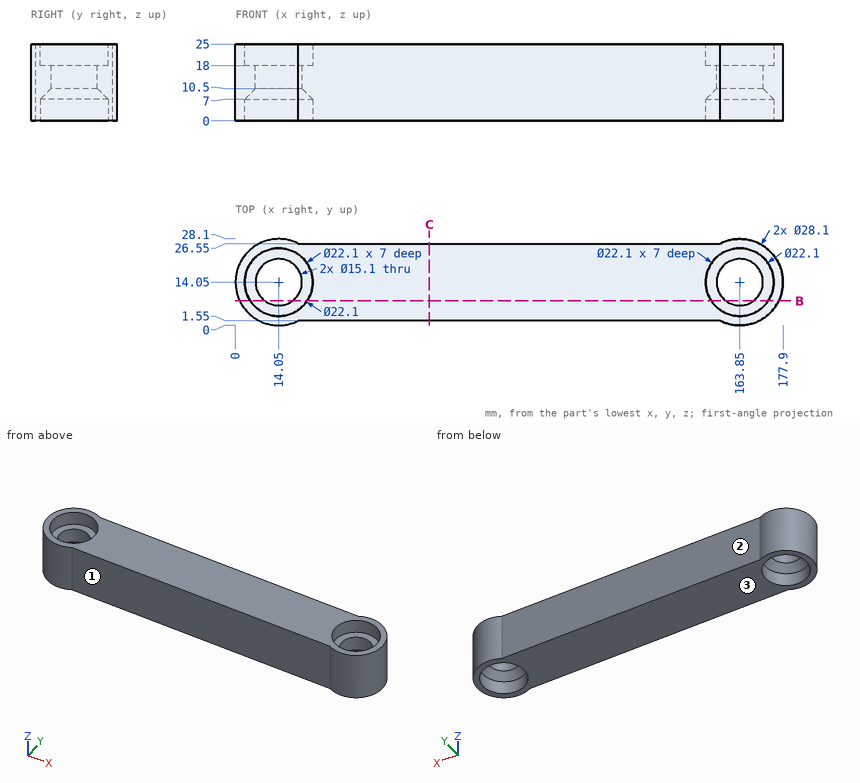
Geometry: see drawing. Coordinates: mm, zero at the bounding-box minimum. Round coordinates to 2 decimals unless told otherwise and drop trailing zeros. Loops run counter-clockwise (first coordinate to the right, second up) from the corner with the lowest first, then second, coordinate; pieces in that order, holes last. Notation, with made-up numbers: (84, 58) - (117, 58) arc R15 cw to (117, 79) - close; hole circle Ø10 at (46, -19.5). An arc over 180 degrees is marked (long way). Write item = value, one per line. Start each with the question number.
(1) Pull-direction query (X, two-part tool) for the marked faces 1, 2 and 3; classes: +X half, -X half, draft (parallel to the pull), parting line (faces both ways), or undercut.
(2) Ray query, line 1 along X through (y, z) = (14.05, 1.5); line 2 along X through (y, z) = (20.25, 13.25); line 3 along Y through (x, z) = (14.05, 15.75). Return the intervals inside material, ascending. Write a range as from..to.
(3) Section query C-C, the plane x = 63. Output: boundary loops of the cut face in (y, z).
(4) Pin query (flat end, axial travel): pin 1 (11 mm diameter, centred on x = 166.5, y = 14, fed in from -Z); pin 2 (5 mm diameter, centred on x = 140, z = 4, fed in from +Y); pin 3 (1.5 mm diameter, centred on x = 47, z = 17, fed in from -Y). Return the tip coordinate at first contact, or that it passes through.
(5) Section query B-B, the plane y = 8. State how many separate pieces and enclosed holes the cut face has, plus the area to 3 significant figures.
Conclusion:
q1.face_1 = undercut
q1.face_2 = undercut
q1.face_3 = draft
q2.line_1 = 0..3, 25.1..152.8, 174.9..177.9
q2.line_2 = 1.44..9.74, 18.36..159.54, 168.16..176.46
q2.line_3 = 0..6.5, 21.6..28.1
q3.outline = (1.55, 0) - (26.55, 0) - (26.55, 25) - (1.55, 25) - close
q4.pin_1 = 9.9
q4.pin_2 = 26.55
q4.pin_3 = 1.55
q5.separate_pieces = 3
q5.enclosed_holes = 0
q5.area = 3,630 mm2
